Verification items for the finished model (mm, model axes). Face numbers are marked on the shaded views. A direction names the side the tool comes from. Give positions to 0.01 mm unless a question says otherwise; leave off trailing zeros. Write each loop counter-clockwise with the first axis right and the second up, starting at its lowest first coordinate (ties: lowest second). Pieces come first, ordered by that corner, then holes.
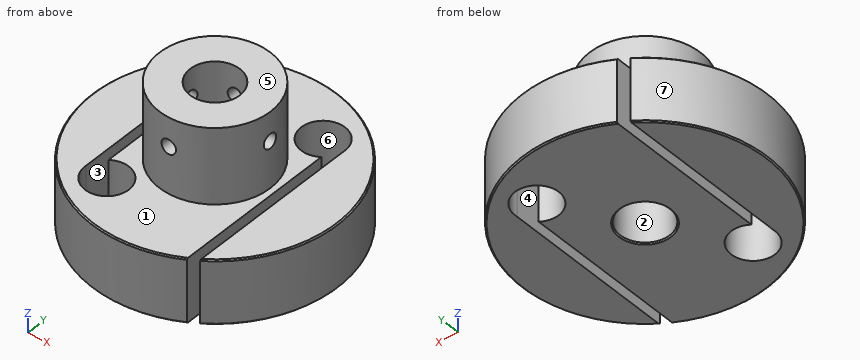
from build123d import *

# Parameters (mm, degrees)
ESQUISSE1_R                               = 21
BOSS_EXTRU_1_DEPTH                        = 11
ESQUISSE2_R                               = 9.5
BOSS_EXTRU_2_DEPTH                        = 13
ESQUISSE3_R                               = 4.25
ENL_V_MAT_EXTRU_1_DEPTH                   = 25
ESQUISSE4_R                               = 3.75
ENL_V_MAT_EXTRU_2_DEPTH                   = 12
ESQUISSE5_W                               = 1.5
ESQUISSE5_H                               = 31.997947006
ESQUISSE5_H_2                             = 31.644558259
ENL_V_MAT_EXTRU_3_DEPTH                   = 12
TROU_POUR_TARAUDAGE_POUR_TROU_TARAUD_M3_D = 2.5
TROU_POUR_TARAUDAGE_POUR_TROU_TARAUD_2_D  = 2.5
CHANFREIN1_SIZE                           = 0.2


with BuildPart() as part:
    # Esquisse1 → Boss.-Extru.1 (new body)
    with BuildSketch(Plane.XY):
        Circle(ESQUISSE1_R)
    extrude(amount=BOSS_EXTRU_1_DEPTH)

    # Esquisse2 → Boss.-Extru.2 (add)
    with BuildSketch(Plane.XY.offset(11)):
        Circle(ESQUISSE2_R)
    extrude(amount=BOSS_EXTRU_2_DEPTH)

    # Esquisse3 → Enlèv. mat.-Extru.1 (cut, through all)
    with BuildSketch(Plane.XY.offset(24)):
        Circle(ESQUISSE3_R)
    extrude(amount=-ENL_V_MAT_EXTRU_1_DEPTH, mode=Mode.SUBTRACT)

    # Esquisse4 → Enlèv. mat.-Extru.2 (cut, through all)
    with BuildSketch(Plane.XY.offset(11)):
        with Locations((8.25, 12.227019261)):
            Circle(ESQUISSE4_R)
        with Locations((-8.25, -12.227019261)):
            Circle(ESQUISSE4_R)
    extrude(amount=-ENL_V_MAT_EXTRU_2_DEPTH, mode=Mode.SUBTRACT)

    # Esquisse5 → Enlèv. mat.-Extru.3 (cut, through all)
    with BuildSketch(Plane.XY.offset(11)):
        with Locations((-11.244697488, 3.971304994)):
            Rectangle(ESQUISSE5_W, ESQUISSE5_H)
        with Locations((11.228919753, -3.198198825)):
            Rectangle(ESQUISSE5_W, ESQUISSE5_H_2)
    extrude(amount=-ENL_V_MAT_EXTRU_3_DEPTH, mode=Mode.SUBTRACT)

    # Trou pour taraudage pour trou taraud_ M3 (through all)
    with Locations(Plane(origin=(0, 10, 0), x_dir=(1, 0, 0), z_dir=(0, 1, 0))):
        with Locations((0, -19)):
            Hole(TROU_POUR_TARAUDAGE_POUR_TROU_TARAUD_M3_D / 2)

    # Trou pour taraudage pour trou taraud 2 (through all)
    with Locations(Plane(origin=(10, 0, 0), x_dir=(0, 0, -1), z_dir=(1, 0, 0))):
        with Locations((-19, 0)):
            Hole(TROU_POUR_TARAUDAGE_POUR_TROU_TARAUD_2_D / 2)

    # Chanfrein1
    chanfrein1_edges = [part.edges().sort_by_distance(p)[0] for p in [
        (-4.25, 0, 0),
        (-17.734235345, -11.24708392, 0),
        (-17.734235345, -11.24708392, 11),
        (17.734504383, 11.246659695, 0),
        (17.734504383, 11.246659695, 11),
    ]]
    chamfer(chanfrein1_edges, length=CHANFREIN1_SIZE)


solid = part.part
Item 1: Set-up check for the marked faces 1, 2, 3 and 4: record each of +Z, -Z, +X, -X, +Y, -Y from which the full face is reachable in a straight line by a thin tool's end or side.
Answer key:
face 1: +Z
face 2: +Z, -Z
face 3: +Z, -Z, +Y
face 4: +Z, -Z, -Y
Item 2: Sectioned sample at B-B on x = 0. Record the cut outline in (y, z), then the cut area to 3 significant figures.
Answer key:
outline: (-21, 0.2) - (-20.8, 0) - (-4.45, 0) - (-4.25, 0.2) - (-4.25, 17.75) - (-9.5, 17.75) - (-9.5, 11) - (-20.8, 11) - (-21, 10.8) - close; (-9.5, 20.25) - (-4.25, 20.25) - (-4.25, 24) - (-9.5, 24) - close; (4.25, 0.2) - (4.45, 0) - (20.8, 0) - (21, 0.2) - (21, 10.8) - (20.8, 11) - (9.5, 11) - (9.5, 17.75) - (4.25, 17.75) - close; (4.25, 20.25) - (9.5, 20.25) - (9.5, 24) - (4.25, 24) - close
area: 479 mm2
Item 3: Sectioned sample at A-A on y = 0. State how many separate pieces and enclosed holes the cut face has, then the cut area to 3 significant figures.
Answer key:
separate pieces: 6
enclosed holes: 0
area: 446 mm2
Item 4: Scan lines: line 1 along Z through (x, y) = (0, 7.3); line 2 along X through (y, z) = (-10, 10.5); line 3 along X through (y, z) = (15, 3). Record each from-to range of solid material in increasing order.
Answer key:
line 1: z = 0 to 17.75, 20.25 to 24
line 2: x = -18.47 to -11.99, -5.23 to 10.48, 11.98 to 18.47
line 3: x = -14.7 to -11.99, -10.49 to 5.73, 10.77 to 14.7
Item 5: Sectioned sample at C-C on z = 5. Record the cut outline in (x, y).
Answer key:
outline: (-11.99, -12.03) - (-11.99, 17.24) arc R21 ccw to (10.48, -18.2) - (10.48, 9.21) arc R3.75 cw (long way) to (11.98, 11.83) - (11.98, -17.25) arc R21 ccw to (-10.49, 18.19) - (-10.49, -9.22) arc R3.75 cw (long way) to start; hole circle Ø8.5 at (0, 0)
Item 6: Release check for a two-part mould opening along Y. For the marked faces 5, 6 and 7 record: released by +Y, released by -Y, zero draft, split by the parting line, or undercut.
Answer key:
face 5: zero draft
face 6: undercut
face 7: split by the parting line
Item 7: Sectioned sample at D-D on z = 19. Record the cut outline in (x, y).
Answer key:
outline: (-9.42, -1.25) arc R9.5 ccw to (-1.25, -9.42) - (-1.25, -4.06) arc R4.25 cw to (-4.06, -1.25) - close; (-9.42, 1.25) - (-4.06, 1.25) arc R4.25 cw to (-1.25, 4.06) - (-1.25, 9.42) arc R9.5 ccw to start; (1.25, -9.42) arc R9.5 ccw to (9.42, -1.25) - (4.06, -1.25) arc R4.25 cw to (1.25, -4.06) - close; (1.25, 4.06) arc R4.25 cw to (4.06, 1.25) - (9.42, 1.25) arc R9.5 ccw to (1.25, 9.42) - close
Item 8: Depth check by flat-ended pin: pin 1 (3 mm diameter, centred on y = 0, z = 19, fed in from +X); pin 2 (9 mm diameter, centred on y = -10, z = 3, fed in from +X); pin 3 (4 mm diameter, centred on y = -3.5, z = 20.5, fed in from +X). Enter the tip coordinate at first touch or a pass-through.
Answer key:
pin 1: stops at x = 9.5
pin 2: stops at x = 20.27
pin 3: stops at x = 9.38
